Work out the finished part from the listing and answer in its coordinate system (mm). A direction names the side the tool comes from. Coordinates: 2 decimals unless noted, no trailing zeros. Order: outer loops, then holes, each group sorted by start corner. A loop starts at its lowest first (then second) coordinate and runs counter-clockwise, first axis right, second up. Notation, with made-up numbers: M 88.25,84.25 L 139.25,84.25 A27 cw 139.25,105.25 Z; hole C 81.5,15 d4. An arc over 180 degrees is marked long. Use a Markdown table: item, result. Add a question column.
from build123d import *

# Parameters (mm, degrees)
SKETCH1_R           = 0.955
BOSS_EXTRUDE1_DEPTH = 2.35


with BuildPart() as part:
    # Sketch1 → Boss-Extrude1 (new body)
    with BuildSketch(Plane.XY):
        with BuildLine():
            ThreePointArc((31.089190509, -0.00961289), (28.777823425, -0.762116774), (27.131493603, -2.550489779))
            ThreePointArc((27.131493603, -2.550489779), (26.201203233, -1.937982234), (25.205610954, -1.438580913))
            ThreePointArc((25.205610954, -1.438580913), (25.931222497, 0.881369039), (25.427226435, 3.259323592))
            ThreePointArc((25.427226435, 3.259323592), (25.075169864, 3.358604023), (24.720639715, 3.448652933))
            ThreePointArc((24.720639715, 3.448652933), (23.095189045, 1.641281911), (22.563612099, -0.730659454))
            ThreePointArc((22.563612099, -0.730659454), (21.451703233, -0.665357545), (20.339794367, -0.730659454))
            ThreePointArc((20.339794367, -0.730659454), (19.80821742, 1.641281911), (18.182766751, 3.448652933))
            ThreePointArc((18.182766751, 3.448652933), (17.828236601, 3.358604023), (17.47618003, 3.259323592))
            ThreePointArc((17.47618003, 3.259323592), (16.972183969, 0.881369039), (17.697795512, -1.438580913))
            ThreePointArc((17.697795512, -1.438580913), (16.702203233, -1.937982234), (15.771912863, -2.550489779))
            ThreePointArc((15.771912863, -2.550489779), (14.12558304, -0.762116774), (11.814215957, -0.00961289))
            ThreePointArc((11.814215957, -0.00961289), (11.552208296, -0.264862608), (11.296958578, -0.526870269))
            ThreePointArc((11.296958578, -0.526870269), (12.049462462, -2.838237352), (13.837835467, -4.484567174))
            ThreePointArc((13.837835467, -4.484567174), (13.225327922, -5.414857545), (12.725926601, -6.410449824))
            ThreePointArc((12.725926601, -6.410449824), (10.40597665, -5.684838281), (8.028022096, -6.188834342))
            ThreePointArc((8.028022096, -6.188834342), (7.928741665, -6.540890913), (7.838692755, -6.895421063))
            ThreePointArc((7.838692755, -6.895421063), (9.646063777, -8.520871732), (12.018005142, -9.052448679))
            ThreePointArc((12.018005142, -9.052448679), (11.952703233, -10.164357545), (12.018005142, -11.276266411))
            ThreePointArc((12.018005142, -11.276266411), (9.646063777, -11.807843357), (7.838692755, -13.433294027))
            ThreePointArc((7.838692755, -13.433294027), (7.928741665, -13.787824176), (8.028022096, -14.139880747))
            ThreePointArc((8.028022096, -14.139880747), (10.40597665, -14.643876808), (12.725926601, -13.918265265))
            ThreePointArc((12.725926601, -13.918265265), (13.225327922, -14.913857545), (13.837835467, -15.844147915))
            ThreePointArc((13.837835467, -15.844147915), (12.049462462, -17.490477737), (11.296958578, -19.80184482))
            ThreePointArc((11.296958578, -19.80184482), (11.552208296, -20.063852481), (11.814215957, -20.3191022))
            ThreePointArc((11.814215957, -20.3191022), (14.12558304, -19.566598315), (15.771912863, -17.77822531))
            ThreePointArc((15.771912863, -17.77822531), (16.702203233, -18.390732855), (17.697795512, -18.890134176))
            ThreePointArc((17.697795512, -18.890134176), (16.972183969, -21.210084128), (17.47618003, -23.588038682))
            ThreePointArc((17.47618003, -23.588038682), (17.828236601, -23.687319113), (18.182766751, -23.777368023))
            ThreePointArc((18.182766751, -23.777368023), (19.80821742, -21.969997001), (20.339794367, -19.598055636))
            ThreePointArc((20.339794367, -19.598055636), (21.451703233, -19.663357545), (22.563612099, -19.598055636))
            ThreePointArc((22.563612099, -19.598055636), (23.095189045, -21.969997001), (24.720639715, -23.777368023))
            ThreePointArc((24.720639715, -23.777368023), (25.075169864, -23.687319113), (25.427226435, -23.588038682))
            ThreePointArc((25.427226435, -23.588038682), (25.931222497, -21.210084128), (25.205610954, -18.890134176))
            ThreePointArc((25.205610954, -18.890134176), (26.201203233, -18.390732855), (27.131493603, -17.77822531))
            ThreePointArc((27.131493603, -17.77822531), (28.777823425, -19.566598315), (31.089190509, -20.3191022))
            ThreePointArc((31.089190509, -20.3191022), (31.351198169, -20.063852481), (31.606447888, -19.80184482))
            ThreePointArc((31.606447888, -19.80184482), (30.853944004, -17.490477737), (29.065570998, -15.844147915))
            ThreePointArc((29.065570998, -15.844147915), (29.678078543, -14.913857545), (30.177479864, -13.918265265))
            ThreePointArc((30.177479864, -13.918265265), (32.497429816, -14.643876808), (34.87538437, -14.139880747))
            ThreePointArc((34.87538437, -14.139880747), (34.974664801, -13.787824176), (35.064713711, -13.433294027))
            ThreePointArc((35.064713711, -13.433294027), (33.257342689, -11.807843357), (30.885401324, -11.276266411))
            ThreePointArc((30.885401324, -11.276266411), (30.950703233, -10.164357545), (30.885401324, -9.052448679))
            ThreePointArc((30.885401324, -9.052448679), (33.257342689, -8.520871732), (35.064713711, -6.895421063))
            ThreePointArc((35.064713711, -6.895421063), (34.974664801, -6.540890913), (34.87538437, -6.188834342))
            ThreePointArc((34.87538437, -6.188834342), (32.497429816, -5.684838281), (30.177479864, -6.410449824))
            ThreePointArc((30.177479864, -6.410449824), (29.678078543, -5.414857545), (29.065570998, -4.484567174))
            ThreePointArc((29.065570998, -4.484567174), (30.853944004, -2.838237352), (31.606447888, -0.526870269))
            ThreePointArc((31.606447888, -0.526870269), (31.351198169, -0.264862608), (31.089190509, -0.00961289))
        make_face()
        with Locations((21.451703233, -10.164357545)):
            Circle(SKETCH1_R, mode=Mode.SUBTRACT)
    extrude(amount=BOSS_EXTRUDE1_DEPTH)


solid = part.part
(1) A cutting plane is placed at D-D on y = -7.25. Write down the section's boundary in (x, z), plus the area to 3 significant figures.
(2) Which of the six approach directions +Z, -Z, +X, -X, +Y, -Y give full straight-line access (tool end or side, diameter ignored) to faces 1 (the cylindrical face through (28.81, -0.74, 1.16)), 2 (the cylindrical face through (25.93, 0.85, 1.16))?
(3) Straight lines are drawn through the part: line 1 (X direction, y = -1.75, z = 0.7); line 2 (Y direction, x = 30.25, z = 1.6); line 3 (X direction, y = -1.5, z = 1.2). For each, find the intervals that lie inside material, in ascending order.
(4) A cutting plane is placed at A-A on x = 32.5. Write down the section's boundary in (y, z), plus the area to 3 significant figures.
(5) A cutting plane is placed at B-B on y = -18.5. Write down the section's boundary in (x, z).
(6) A cutting plane is placed at C-C on y = 1.5. Write down the section's boundary in (x, z), plus the area to 3 significant figures.
(7) Given P1, Ø1, axis at y = -10, z = 2, coming from the -X side, flat-ended and moving along its own axis, determine where the tip first touches the part or whether it passes through.
From the geometry:
| question | item | result |
|---|---|---|
| 1 | outline | M 8.1,0 L 34.81,0 L 34.81,2.35 L 8.1,2.35 Z |
| 1 | area | 62.8 mm2 |
| 2 | face 1 | +Z, -Z, +Y |
| 2 | face 2 | +Z, -Z |
| 3 | line 1 | x = 11.53 to 15.24, 17.04 to 25.86, 27.67 to 31.37 |
| 3 | line 2 | y = -20.19 to -16.73, -13.96 to -6.37, -3.6 to -0.13 |
| 3 | line 3 | x = 11.46 to 15.02, 17.56 to 25.35, 27.89 to 31.45 |
| 4 | outline | M -14.64,0 L -11.5,0 L -11.5,2.35 L -14.64,2.35 Z; M -8.83,0 L -5.68,0 L -5.68,2.35 L -8.83,2.35 Z |
| 4 | area | 14.8 mm2 |
| 5 | outline | M 11.56,0 L 15.3,0 L 15.3,2.35 L 11.56,2.35 Z; M 16.9,0 L 26.01,0 L 26.01,2.35 L 16.9,2.35 Z; M 27.6,0 L 31.35,0 L 31.35,2.35 L 27.6,2.35 Z |
| 6 | outline | M 16.98,0 L 19.88,0 L 19.88,2.35 L 16.98,2.35 Z; M 23.03,0 L 25.92,0 L 25.92,2.35 L 23.03,2.35 Z |
| 6 | area | 13.6 mm2 |
| 7 | P1 | stops at x = 11.95 |
